For this review, take the finished solid that the model builds, in its own axes (mm). Give positions to 0.01 mm unless a question says otherwise; leave off trailing zeros. Write each loop counter-clockwise with the first axis right and the second up, starting at its lowest first coordinate (ties: lowest second). Pieces come first, ordered by that corner, then holes. Notation, with made-up numbers: (15.25, 28) -> (52.25, 28) arc R22 ccw to (52.25, 65) -> close; hole circle Ø2 at (-10, 23). An arc over 180 degrees is marked (long way). Write item = value, one per line.
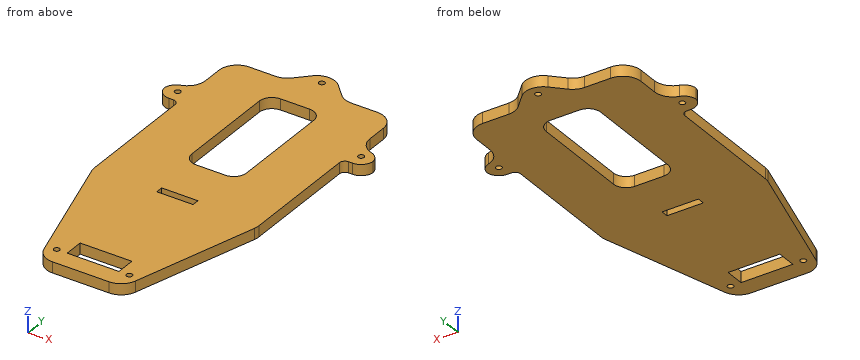
```python
from build123d import *

# Parameters (mm, degrees)
ESBO_O1_R                = 1.6
ESBO_O1_W                = 28.5
ESBO_O1_H                = 10.6
ESBO_O1_W_2              = 30
ESBO_O1_H_2              = 69.1
ESBO_O1_W_3              = 20
ESBO_O1_H_3              = 4
RESSALTO_EXTRUS_O1_DEPTH = 6
FILETE3_R                = 3
FILETE4_R                = 10
FILETE5_R                = 7
ESBO_O2_R                = 1.6
CORTE_EXTRUS_O1_DEPTH    = 10


with BuildPart() as part:
    # Esboço1 → Ressalto-extrusão1 (new body)
    with BuildSketch(Plane.XY):
        Polygon((-45.25, -56.75), (-23.05952475, -133.85), (23.05952475, -133.85), (45.25, -56.75), (45.25, 13.75), (57.5, 13.75), (57.5, 25.75), (45.25, 25.75), (45.25, 56.75), (16.663333, 56.75), (0, 73.75), (-16.663333, 56.75), (-45.25, 56.75), (-45.25, 25.75), (-57.5, 25.75), (-57.5, 13.75), (-45.25, 13.75), align=None)
        with Locations((0, 63.75)):
            Circle(ESBO_O1_R, mode=Mode.SUBTRACT)
        with Locations((-50.5, 20.75)):
            Circle(ESBO_O1_R, mode=Mode.SUBTRACT)
        with Locations((50.5, 20.75)):
            Circle(ESBO_O1_R, mode=Mode.SUBTRACT)
        with Locations((0, -118.55)):
            Rectangle(ESBO_O1_W, ESBO_O1_H, mode=Mode.SUBTRACT)
        with Locations((0, 7.2)):
            Rectangle(ESBO_O1_W_2, ESBO_O1_H_2, mode=Mode.SUBTRACT)
        with Locations((0, -54.75)):
            Rectangle(ESBO_O1_W_3, ESBO_O1_H_3, mode=Mode.SUBTRACT)
    extrude(amount=RESSALTO_EXTRUS_O1_DEPTH)

    # Filete3
    filete3_edges = [part.edges().sort_by_distance(p)[0] for p in [
        (-45.25, 13.75, 3),
        (45.25, 13.75, 3),
    ]]
    fillet(filete3_edges, radius=FILETE3_R)

    # Filete4
    filete4_edges = [part.edges().sort_by_distance(p)[0] for p in [
        (-45.25, 25.75, 3),
        (-45.25, 56.75, 3),
        (-16.663333, 56.75, 3),
        (0, 73.75, 3),
        (16.663333, 56.75, 3),
        (45.25, 56.75, 3),
        (45.25, 25.75, 3),
        (45.25, -56.75, 3),
        (23.05952475, -133.85, 3),
        (-23.05952475, -133.85, 3),
        (-45.25, -56.75, 3),
    ]]
    fillet(filete4_edges, radius=FILETE4_R)

    # Filete5
    # the kernel refuses this fillet: 7 mm, written as the material it adds along each edge
    with BuildSketch(Plane(origin=(-15, -27.35, 0), x_dir=(1, 0, 0), z_dir=(0, 0, 1)), Plane(origin=(15, 41.75, 0), x_dir=(-1, 0, 0), z_dir=(0, 0, 1)), Plane(origin=(-15, 41.75, 0), x_dir=(0, -1, 0), z_dir=(0, 0, 1))) as filete5_piece_1:
        with BuildLine():
            CenterArc((FILETE5_R, FILETE5_R), FILETE5_R, 180, 90)
            Line((0, FILETE5_R), (0, 0))
            Line((0, 0), (FILETE5_R, 0))
        make_face()
    extrude(amount=6)
    with BuildSketch(Plane(origin=(15, -27.35, 0), x_dir=(-1, 0, 0), z_dir=(0, 0, 1))) as filete5_piece_2:
        with BuildLine():
            CenterArc((FILETE5_R, -FILETE5_R), FILETE5_R, 90, 90)
            Line((0, -FILETE5_R), (0, 0))
            Line((0, 0), (FILETE5_R, 0))
        make_face()
    extrude(amount=6)
    # the kernel refuses this fillet: 7 mm, written as the material it takes off along each edge
    with BuildSketch(Plane(origin=(57.5, 13.75, -17.5), x_dir=(-1, 0, 0), z_dir=(0, 0, 1))) as filete5_2_piece_1:
        with BuildLine():
            CenterArc((FILETE5_R, -FILETE5_R), FILETE5_R, 90, 90)
            Line((0, -FILETE5_R), (0, 0))
            Line((0, 0), (FILETE5_R, 0))
        make_face()
    extrude(amount=41, mode=Mode.SUBTRACT)
    with BuildSketch(Plane(origin=(57.5, 25.75, -15.807283357), x_dir=(0, -1, 0), z_dir=(0, 0, 1))) as filete5_2_piece_2:
        with BuildLine():
            CenterArc((6.322913343, -7), FILETE5_R, 90, 73.774899865)
            Line((-0.398286269, -5.044117647), (-1.07040623, -4.848529412))
            ThreePointArc((-1.07040623, -4.848529412), (-0.7, -2.25), (-0.7, 0))
            Line((-0.7, 0), (0, 0.7))
            Line((0, 0.7), (6.322913343, 0.7))
            Line((6.322913343, 0.7), (6.322913343, 0))
        make_face()
    extrude(amount=37.614566715, mode=Mode.SUBTRACT)
    with BuildSketch(Plane(origin=(-57.5, 13.75, -17.5), x_dir=(1, 0, 0), z_dir=(0, 0, 1))) as filete5_2_piece_3:
        with BuildLine():
            CenterArc((FILETE5_R, FILETE5_R), FILETE5_R, 180, 90)
            Line((0, FILETE5_R), (0, 0))
            Line((0, 0), (FILETE5_R, 0))
        make_face()
    extrude(amount=41, mode=Mode.SUBTRACT)
    with BuildSketch(Plane(origin=(-57.5, 25.75, -15.807283357), x_dir=(0, -1, 0), z_dir=(0, 0, 1))) as filete5_2_piece_4:
        with BuildLine():
            CenterArc((6.322913343, 7), FILETE5_R, 196.225100135, 73.774899865)
            Line((-0.398286269, 5.044117647), (-1.07040623, 4.848529412))
            ThreePointArc((-1.07040623, 4.848529412), (-0.7, 2.25), (-0.7, 0))
            Line((-0.7, 0), (0, -0.7))
            Line((0, -0.7), (6.322913343, -0.7))
            Line((6.322913343, -0.7), (6.322913343, 0))
        make_face()
    extrude(amount=37.614566715, mode=Mode.SUBTRACT)

    # Esboço2 → Corte-extrusão1 (cut)
    with BuildSketch(Plane.XY.offset(6)):
        with Locations((-20, -123.85)):
            Circle(ESBO_O2_R)
        with Locations((20, -123.85)):
            Circle(ESBO_O2_R)
    extrude(amount=-CORTE_EXTRUS_O1_DEPTH, mode=Mode.SUBTRACT)


solid = part.part
```
(1) Take a section at A-A (x = -4.5). Write out the cut boundary in (y, z).
Answers below:
outline = (-133.85, 0) -> (-123.85, 0) -> (-123.85, 6) -> (-133.85, 6) -> close; (-113.25, 0) -> (-56.75, 0) -> (-56.75, 6) -> (-113.25, 6) -> close; (-52.75, 0) -> (-27.35, 0) -> (-27.35, 6) -> (-52.75, 6) -> close; (41.75, 0) -> (68.39, 0) -> (68.39, 6) -> (41.75, 6) -> close
(2) Take a section at B-B (z = 1.05). Count the separate pieces of the cut face and the enclosed holes in it, plus the area to 3 significant figures.
Answers below:
separate_pieces = 1
enclosed_holes = 8
area = 13,600 mm^2
(3) For pin 1 (3 mm diameter, centred on y = -54.5, z = 4, fed in from -X); pin 2 (1.8 mm diameter, centred on x = 49, z = 2, fed in from -Y); pin 3 (3 mm diameter, centred on y = -17.5, z = 4, fed in from +X); pin 4 (3 mm diameter, centred on x = 20, y = -123.85, fed in from +Z), all flat-tipped, find the tip position at first contact; note any pin that passes through.
Answers below:
pin_1 = -45.25
pin_2 = 13.75
pin_3 = 45.25
pin_4 = through
(4) Take a section at D-D (x = -38.5). Write out the cut boundary in (y, z), plus the area to 3 significant figures.
Answers below:
outline = (-80.2, 0) -> (56.21, 0) -> (56.21, 6) -> (-80.2, 6) -> close
area = 818 mm^2
(5) To check wall thickness, follow probe 1 along Y at (x, z) = (0, 4.6); probe 2 along X at (y, z) = (-5.5, 0.9); probe 3 along Y at (x, z) = (9.5, 5.55). State the ranges of each line that lie inside material, in increasing order.
Answers below:
probe_1 = -133.85 to -123.85, -113.25 to -56.75, -52.75 to -27.35, 41.75 to 62.15, 65.35 to 69.46
probe_2 = -45.25 to -15, 15 to 45.25
probe_3 = -133.85 to -123.85, -113.25 to -56.75, -52.75 to -27.19, 41.59 to 64.06
(6) Take a section at C-C (y = -98.5). Write out the cut boundary in (x, z), plus the area to 3 significant figures.
Answers below:
outline = (-33.23, 0) -> (33.23, 0) -> (33.23, 6) -> (-33.23, 6) -> close
area = 399 mm^2
